Source: CAD feature listing. Evaluate the final solid. Frame: model axes, mm. A direction names the side the tool comes from. Coordinates: 2 decimals unless noted, no trailing zeros. Loops run counter-clockwise (first coordinate to the right, second up) from the corner with the lowest first, then second, coordinate; pieces in that order, holes last.
Autodesk Inventor part; units mm, degrees
ref_plane "YZ Plane" through (0, 0, 0) normal (1, 0, 0) x (0, 1, 0)
ref_plane "XZ Plane" through (0, 0, 0) normal (0, 1, 0) x (-1, 0, 0)
ref_plane "XY Plane" through (0, 0, 0) normal (0, 0, 1) x (1, 0, 0)
sketch "Эскиз1" plane through (0, 0, 0) normal (0, 0, 1) x (1, 0, 0)
  line L0 (-38, 52.38) -> (38, 52.38) construction
  line L1 (38, 52.38) -> (38, -52.38) construction
  line L2 (38, -52.38) -> (-38, -52.38) construction
  line L3 (-38, -52.38) -> (-38, 52.38) construction
  line L4 (-26.6205, -33.05) -> (26.6205, -33.05) construction
  line L5 (26.6205, -33.05) -> (26.6205, 33.05) construction
  line L6 (26.6205, 33.05) -> (-26.6205, 33.05) construction
  line L7 (-26.6205, 33.05) -> (-26.6205, -33.05) construction
  line L8 (0, 33.05) -> (0, 38.05) construction
  line L9 (0, -33.05) -> (0, -38.05) construction
  line L10 (-38, 38.05) -> (38, 38.05)
  line L11 (38, 38.05) -> (38, -38.05)
  line L12 (38, -38.05) -> (-38, -38.05)
  line L13 (-38, -38.05) -> (-38, 38.05)
  dimension "d0" = 76
  dimension "d1" = 104.76
  dimension "d2" = 53.241
  dimension "d3" = 66.1
  dimension "d4" = 5
  dimension "d5" = 5
extrude "Выдавливание1" add sketch "Эскиз1" along normal blind 5
sketch "Эскиз2" plane through (0, 0, 5) normal (0, 0, 1) x (1, 0, 0)
  line L0 (38, 38.05) -> (38, -38.05)
  line L1 (-38, -38.05) -> (-38, 38.05)
  line L2 (-38, 38.05) -> (-38, -38.05)
  line L3 (-38, -38.05) -> (-42, -38.05)
  line L4 (38, 38.05) -> (42, 38.05)
  line L5 (42, -38.05) -> (42, 38.05)
  line L6 (-42, 38.05) -> (-42, -38.05)
  line L7 (-38, -38.05) -> (-38, 38.05)
  line L8 (38, 38.05) -> (-38, 38.05)
  line L9 (38, 38.05) -> (38, -38.05)
  line L10 (42, 38.05) -> (38, 38.05)
  line L11 (-38, 38.05) -> (-42, 38.05)
  line L12 (-42, -38.05) -> (-38, -38.05)
  line L13 (38, -38.05) -> (42, -38.05)
  point P0 (0, 0)
  dimension "d8" = 4
  dimension "d9" = 4
extrude "Выдавливание2" add sketch "Эскиз2" along normal blind 24 and the other way blind 5
sketch "Эскиз3" plane through (0, 0, 29) normal (0, 0, 1) x (1, 0, 0)
  line L0 (38, 38.05) -> (38, -38.05)
  line L1 (38, -38.05) -> (42, -38.05)
  line L2 (42, -38.05) -> (42, 38.05)
  line L3 (42, 38.05) -> (38, 38.05)
  line L4 (42, 9.5) -> (38, 9.5)
  line L5 (38, 9.5) -> (38, -9.5)
  line L6 (38, -9.5) -> (42, -9.5)
  line L7 (42, -9.5) -> (42, 9.5)
  line L8 (42, 9.5) -> (38, -9.5) construction
  line L9 (38, 9.5) -> (42, -9.5) construction
  line L10 (0, 0) -> (0, -84) construction
  line L11 (-42, 9.5) -> (-38, 9.5)
  line L12 (-38, -9.5) -> (-42, -9.5)
  line L13 (-38, 9.5) -> (-38, -9.5) construction
  line L14 (-38, 38.05) -> (-38, -38.05) construction
  line L15 (-42, 9.5) -> (-42, -9.5) construction
  line L16 (-42, 38.05) -> (-42, -38.05) construction
  line L17 (-38, 9.5) -> (-38, -9.5)
  line L18 (-42, -9.5) -> (-42, 9.5)
  point P0 (40, 0)
  dimension "d14" = 4
  dimension "d15" = 19
extrude "Выдавливание3" cut sketch "Эскиз3" against normal up to surface (24 mm away) contours L4 L2 L6 L0 | L11 L17 L12 L18
sketch "Эскиз4" plane through (-42, 38.05, 0) normal (0, 1, 0) x (1, 0, 0)
  line L0 (0, 0) -> (84, 0)
  line L1 (0, 0) -> (0, -29)
  line L2 (4, -29) -> (0, -29)
  line L3 (4, -29) -> (4, -5)
  line L4 (80, -5) -> (4, -5)
  line L5 (80, -29) -> (80, -5)
  line L6 (84, -29) -> (80, -29)
  line L7 (84, 0) -> (84, -29)
  point P0 (42, 0)
extrude "Выдавливание4" cut sketch "Эскиз4" against normal blind 29
sketch "Эскиз5" plane through (0, 0, 29) normal (0, 0, 1) x (1, 0, 0)
  line L0 (-38, -9.5) -> (-42, -9.5)
  line L1 (-42, -9.5) -> (-42, -38.05)
  line L2 (-42, -38.05) -> (-38, -38.05)
  line L3 (-38, -38.05) -> (-38, -9.5)
  line L4 (42, -9.5) -> (38, -9.5)
  line L5 (38, -9.5) -> (38, -38.05)
  line L6 (38, -38.05) -> (42, -38.05)
  line L7 (42, -38.05) -> (42, -9.5)
  point P0 (0, 0)
extrude "Выдавливание5" add sketch "Эскиз5" along normal blind 12
sketch "Эскиз6" plane through (42, -9.5, 5) normal (1, 0, 0) x (0, 0, -1)
  line L0 (5, 18.55) -> (0, 18.55)
  line L1 (0, 18.55) -> (0, 0)
  line L2 (0, 0) -> (-36, 0)
  line L3 (-36, -28.55) -> (-36, 0)
  line L4 (5, -28.55) -> (-36, -28.55)
  line L5 (5, 18.55) -> (5, -28.55)
  line L6 (-36, -28.55) -> (-36, 0) construction
  line L7 (-36, -14.275) -> (-27, -14.275) construction
  circle A0 centre (-27, -14.275) radius 2
  point P0 (5, 9.5)
  dimension "d22" = 9
  dimension "d23" = 4
extrude "Выдавливание6" cut sketch "Эскиз6" against normal up to surface (84 mm away) contours A0
properties part number "Ard for BR"
Q1. Material intervals for line 1 along X through (y, z) = (-31, 19.5); line 2 along Y through (x, z) = (-39.1, 32) (3 decimals); line 3 along Z through (x, y) = (9, 5), sorted ascending.
Q2. Section query A-A on z = 32. Return the cut outline in (x, y) (3 decimals).
Q3. Section query B-B on y = -11.5. Return the cut outline in (x, z).
Q4. Section query D-D on x = -27.5. Return the cut outline in (y, z), then the cut area to 4 significant figures.
Q5. Section query C-C on z = 23.5. Return the cut outline in (x, y).
Q6. First-contact query: pin 1 Ø23.5 at (x, y) = (18.5, -12.5) entering from +Z; pin 2 Ø4.5 at (x, z) = (39.5, 28.5) entering from +Y. Flat tips, straight axial feed; report the tip coordinate or a pass-through.
Q7. Reachability of faces 1 (the flat face through (-40, -9.5, 23)), 2 (the flat face through (40, -24, 41)), 3 (the flat face through (-38, -24, 23)) from +Z, -Z, +X, -X, +Y, -Y: full face, straight path, thin tool, end or side. Return the list, or none.
Q8. Draft query along Y for faces 4 (the flat face through (38, -24, 23)), 5 (the flat face through (-1, 9.05, 2)), 6 (the cylindrical face through (40.03, -24.54, 30.15)). Return one class per face: released by +Y, released by -Y, zero draft, split by the parting line, or undercut.
Resolved:
1. line 1: x = -42 to -38, 38 to 42
1. line 2: y = -38.05 to -25.775, -21.775 to -9.5
1. line 3: z = 0 to 5
2. outline: (-42, -38.05) - (-38, -38.05) - (-38, -25.775) - (-42, -25.775) - close; (-42, -21.775) - (-38, -21.775) - (-38, -9.5) - (-42, -9.5) - close; (38, -38.05) - (42, -38.05) - (42, -25.775) - (38, -25.775) - close; (38, -21.775) - (42, -21.775) - (42, -9.5) - (38, -9.5) - close
3. outline: (-42, 0) - (42, 0) - (42, 41) - (38, 41) - (38, 5) - (-38, 5) - (-38, 41) - (-42, 41) - close
4. outline: (-38.05, 0) - (9.05, 0) - (9.05, 5) - (-38.05, 5) - close
4. area: 235.5 mm2
5. outline: (-42, -38.05) - (-38, -38.05) - (-38, -9.5) - (-42, -9.5) - close; (38, -38.05) - (42, -38.05) - (42, -9.5) - (38, -9.5) - close
6. pin 1: stops at z = 5
6. pin 2: stops at y = -9.5
7. face 1: +Z, +X, -X, +Y
7. face 2: +Z, +X, -X, +Y, -Y
7. face 3: +Z, +Y, -Y
8. face 4: zero draft
8. face 5: released by +Y
8. face 6: undercut
